Read the model definition and answer for the solid it produces. Units are mm, in the model's axes. Face numbers are marked on the shaded views. A direction names the side the tool comes from. Round coordinates to 2 decimals unless told otherwise and drop trailing zeros. Order: outer loops, then holes, each group sorted by start corner. A loop starts at its lowest first (then second) coordinate and runs counter-clockwise, first axis right, second up. Notation, with made-up numbers: (85, 31) -> (130, 31) arc R18 cw to (130, 37) -> close; hole circle Ø11 at (-18.75, -28.5). An arc over 180 degrees is marked (long way). One line per item, written item: value. Start each with the question number.
1. Section A-A (z = 126.5) is taken. Give the vertices of the cut face in (x, y).
2. Section C-C (z = 105) is taken. Give the vertices of the cut face in (x, y), then the cut area to 3 significant figures.
3. For the marked faces 1 and 2, determine the directions among +Z, -Z, +X, -X, +Y, -Y from which every point of the face is accessible in a straight line to the end or side of a thin tool.
4. Section D-D (y = -7.5) is taken. Give the vertices of the cut face in (x, z), then the cut area to 3 significant figures.
5. Section B-B (x = 71) is taken. Give the vertices of the cut face in (y, z), then the cut area to 3 significant figures.
6. Consider line 1 (Z direction, x = 67, y = 0.75); line 2 (Y direction, x = 59.5, z = 125); line 3 (X direction, y = -4.25, z = 46.5). Determine where each line is inside the solid, lowest interval first.
7. Flat-ended cylindrical pins translate along their axes: pin 1 Ø5 at (x, z) = (48, 155) entering from -Y; pin 2 Ø4 at (x, z) = (61.5, 40.5) entering from +Y; pin 3 Ø6.5 at (y, z) = (-8.5, 80) entering from +X. Find the tip coordinate at first contact, or state that the pin passes through.
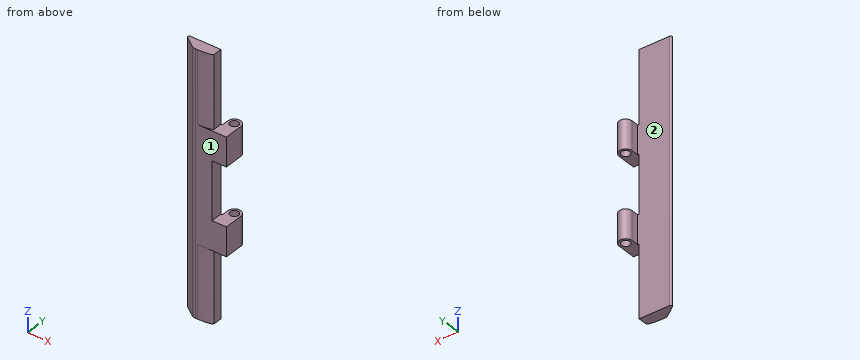
from build123d import *

# Parameters (mm, degrees)
SKETCH1_R           = 3
BOSS_EXTRUDE2_DEPTH = 180
SKETCH3_W           = 10
SKETCH3_H           = 50
CUT_EXTRUDE1_DEPTH  = 32
SKETCH4_W           = 10
SKETCH4_H           = 40
CUT_EXTRUDE2_DEPTH  = 32
FILLET3_R           = 1
FILLET4_R           = 5
FILLET5_SIZE        = 10
FILLET5_SIZE_2      = 2


with BuildPart() as part:
    # Sketch1 → Boss-Extrude2 (new body)
    # profile 1 of 2: a face of its own
    with BuildSketch(Plane.XY):
        with BuildLine():
            Line((75.196634753, -12.063439291), (75.196634753, 0.936560709))
            ThreePointArc((75.196634753, 0.936560709), (70.696634753, 5.436560709), (66.196634753, 0.936560709))
            Line((66.196634753, 0.936560709), (66.196634753, -4.063439291))
            Line((66.196634753, -4.063439291), (66.196634753, -12.063439291))
            Line((66.196634753, -12.063439291), (75.196634753, -12.063439291))
        make_face()
        with Locations(Location((70.696634753, 0.936560709, 0), (0, 0, 180))):
            Circle(SKETCH1_R, mode=Mode.SUBTRACT)
    # profile 2 of 2: a face of its own
    with BuildSketch(Plane.XY):
        with BuildLine():
            Line((41.196634753, -4.063439291), (66.196634753, -4.063439291))
            Line((66.196634753, -4.063439291), (66.196634753, -12.063439291))
            Line((66.196634753, -12.063439291), (52.196634753, -12.063439291))
            ThreePointArc((52.196634753, -12.063439291), (46.632466814, -8.151670207), (41.196634753, -4.063439291))
        make_face()
    extrude(amount=BOSS_EXTRUDE2_DEPTH)

    # Sketch3 → Cut-Extrude1 (cut)
    with BuildSketch(Plane.XZ.offset(12.063439291)):
        with Locations((70.196634753, 155)):
            Rectangle(SKETCH3_W, SKETCH3_H)
        with Locations((70.196634753, 25)):
            Rectangle(SKETCH3_W, SKETCH3_H)
    extrude(amount=-CUT_EXTRUDE1_DEPTH, mode=Mode.SUBTRACT)

    # Sketch4 → Cut-Extrude2 (cut)
    with BuildSketch(Plane(origin=(0, -12.063439291, 0), x_dir=(-1, 0, 0), z_dir=(0, -1, 0))):
        with Locations((-70.196634753, -90)):
            Rectangle(SKETCH4_W, SKETCH4_H)
    extrude(amount=-CUT_EXTRUDE2_DEPTH, mode=Mode.SUBTRACT)

    # Fillet3
    fillet3_edges = [part.edges().sort_by_distance(p)[0] for p in [
        (41.196634753, -4.063439291, 90),
    ]]
    fillet(fillet3_edges, radius=FILLET3_R)

    # Fillet4
    fillet4_edges = [part.edges().sort_by_distance(p)[0] for p in [
        (52.196634753, -12.063439291, 90),
    ]]
    fillet(fillet4_edges, radius=FILLET4_R)

    # Fillet5
    # an asymmetric fillet: 10, 2 mm, written as the material it takes off along each edge
    with BuildSketch(Plane(origin=(65.196634753, -12.063439291, 205), x_dir=(-1, 0, 0), z_dir=(0, 0, -1))) as fillet5_piece_1:
        with BuildLine():
            Bezier((FILLET5_SIZE, 0), (0, 0), (0, FILLET5_SIZE_2), weights=[1, 0.707106781, 1])
            Line((0, FILLET5_SIZE_2), (0, 0))
            Line((0, 0), (FILLET5_SIZE, 0))
        make_face()
    extrude(amount=75, mode=Mode.SUBTRACT)
    with BuildSketch(Plane(origin=(65.196634753, -12.063439291, -25), x_dir=(-1, 0, 0), z_dir=(0, 0, 1))) as fillet5_piece_2:
        with BuildLine():
            Bezier((FILLET5_SIZE, 0), (0, 0), (0, -FILLET5_SIZE_2), weights=[1, 0.707106781, 1])
            Line((0, -FILLET5_SIZE_2), (0, 0))
            Line((0, 0), (FILLET5_SIZE, 0))
        make_face()
    extrude(amount=75, mode=Mode.SUBTRACT)


solid = part.part
Answer:
1. outline: (43.54, -5.86) arc R212.02 ccw to (50.9, -11.18) arc R5 ccw to (53.74, -12.06) -> (75.2, -12.06) -> (75.2, 0.94) arc R4.5 ccw to (66.2, 0.94) -> (66.2, -4.06) -> (44.15, -4.06) arc R1 ccw to start; hole circle Ø6 at (70.7, 0.94)
2. outline: (43.54, -5.86) arc R212.02 ccw to (50.9, -11.18) arc R5 ccw to (53.74, -12.06) -> (65.2, -12.06) -> (65.2, -4.06) -> (44.15, -4.06) arc R1 ccw to start
2. area: 147 mm^2
3. face 1: +Z, -Z, +X, -X, -Y
3. face 2: +Z, -Z, -X, +Y
4. outline: (45.74, 0) -> (65.2, 0) -> (65.2, 50) -> (75.2, 50) -> (75.2, 70) -> (65.2, 70) -> (65.2, 110) -> (75.2, 110) -> (75.2, 130) -> (65.2, 130) -> (65.2, 180) -> (45.74, 180) -> close
4. area: 3,900 mm^2
5. outline: (-12.06, 50) -> (-2.05, 50) -> (-2.05, 70) -> (-12.06, 70) -> close; (-12.06, 110) -> (-2.05, 110) -> (-2.05, 130) -> (-12.06, 130) -> close; (3.92, 50) -> (5.43, 50) -> (5.43, 70) -> (3.92, 70) -> close; (3.92, 110) -> (5.43, 110) -> (5.43, 130) -> (3.92, 130) -> close
5. area: 461 mm^2
6. line 1: 50 to 70, 110 to 130
6. line 2: -12.06 to -4.06
6. line 3: 43.56 to 65.2
7. pin 1: y = -10.9
7. pin 2: y = -4.06
7. pin 3: x = 65.2
